Design review of the part built by this model. Coordinates are the model's own, in mm. Coordinates: 2 decimals unless noted, no trailing zeros. Loops run counter-clockwise (first coordinate to the right, second up) from the corner with the lowest first, then second, coordinate; pieces in that order, holes last. Notation, with made-up numbers: (2, 13) - (13, 13) arc R34 cw to (13, 43) - close; hole circle Ø11 at (31, 0.5). An arc over 180 degrees is marked (long way). One line per question, with ' | ' between items.
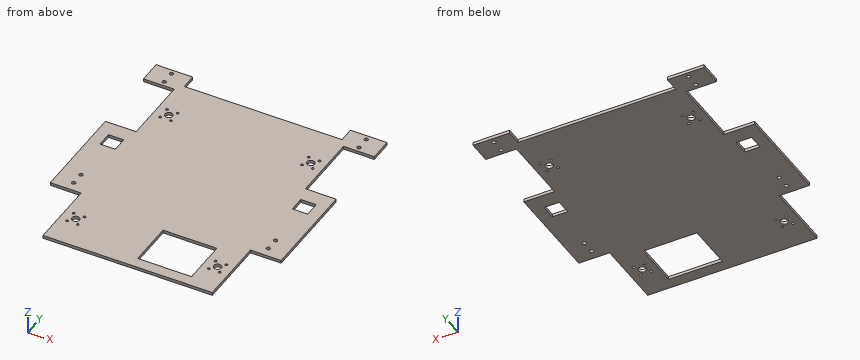
from build123d import *

# Parameters (mm, degrees)
SKETCH_2_R          = 1.65
SKETCH_2_R_2        = 4.9
SKETCH_2_R_3        = 2.5
EXTRUDE_1_DEPTH     = 4
SKETCH_5_W          = 20
SKETCH_5_H          = 20
CUT_EXTRUDE_1_DEPTH = 10
SKETCH_6_W          = 70
SKETCH_6_H          = 60
CUT_EXTRUDE_2_DEPTH = 10


with BuildPart() as part:
    # Sketch 2 → Extrude 1 (new body)
    with BuildSketch(Plane.XY):
        Polygon((40, 0), (260, 0), (260, 90), (300, 90), (300, 220), (260, 220), (260, 310), (300, 310), (300, 340), (252.5, 340), (252.5, 320), (47.5, 320), (47.5, 340), (0, 340), (0, 310), (40, 310), (40, 220), (0, 220), (0, 90), (40, 90), align=None)
        with Locations((50.85, 273)):
            Circle(SKETCH_2_R, mode=Mode.SUBTRACT)
        with Locations((64.85, 273)):
            Circle(SKETCH_2_R, mode=Mode.SUBTRACT)
        with Locations(Location((64.85, 257, 0), (0, 0, 180))):
            Circle(SKETCH_2_R, mode=Mode.SUBTRACT)
        with Locations(Location((50.85, 257, 0), (0, 0, 180))):
            Circle(SKETCH_2_R, mode=Mode.SUBTRACT)
        with Locations((57.8, 265)):
            Circle(SKETCH_2_R_2, mode=Mode.SUBTRACT)
        with Locations((235.15, 257)):
            Circle(SKETCH_2_R, mode=Mode.SUBTRACT)
        with Locations((249.15, 257)):
            Circle(SKETCH_2_R, mode=Mode.SUBTRACT)
        with Locations(Location((242.2, 265, 0), (0, 0, 180))):
            Circle(SKETCH_2_R_2, mode=Mode.SUBTRACT)
        with Locations(Location((235.15, 273, 0), (0, 0, 180))):
            Circle(SKETCH_2_R, mode=Mode.SUBTRACT)
        with Locations(Location((249.15, 273, 0), (0, 0, 180))):
            Circle(SKETCH_2_R, mode=Mode.SUBTRACT)
        with Locations(Location((249.15, 53, 0), (0, 0, 180))):
            Circle(SKETCH_2_R, mode=Mode.SUBTRACT)
        with Locations(Location((235.15, 53, 0), (0, 0, 180))):
            Circle(SKETCH_2_R, mode=Mode.SUBTRACT)
        with Locations((249.15, 37)):
            Circle(SKETCH_2_R, mode=Mode.SUBTRACT)
        with Locations((242.2, 45)):
            Circle(SKETCH_2_R_2, mode=Mode.SUBTRACT)
        with Locations((235.15, 37)):
            Circle(SKETCH_2_R, mode=Mode.SUBTRACT)
        with Locations((50.85, 53)):
            Circle(SKETCH_2_R, mode=Mode.SUBTRACT)
        with Locations((64.85, 53)):
            Circle(SKETCH_2_R, mode=Mode.SUBTRACT)
        with Locations(Location((64.85, 37, 0), (0, 0, 180))):
            Circle(SKETCH_2_R, mode=Mode.SUBTRACT)
        with Locations(Location((57.8, 45, 0), (0, 0, 180))):
            Circle(SKETCH_2_R_2, mode=Mode.SUBTRACT)
        with Locations(Location((50.85, 37, 0), (0, 0, 180))):
            Circle(SKETCH_2_R, mode=Mode.SUBTRACT)
        with Locations((23.5, 333.5)):
            Circle(SKETCH_2_R_3, mode=Mode.SUBTRACT)
        with Locations((23.5, 316.5)):
            Circle(SKETCH_2_R_3, mode=Mode.SUBTRACT)
        with Locations(Location((276.5, 316.5, 0), (0, 0, 180))):
            Circle(SKETCH_2_R_3, mode=Mode.SUBTRACT)
        with Locations(Location((276.5, 333.5, 0), (0, 0, 180))):
            Circle(SKETCH_2_R_3, mode=Mode.SUBTRACT)
        with Locations((23.5, 119.5)):
            Circle(SKETCH_2_R_3, mode=Mode.SUBTRACT)
        with Locations((23.5, 102.5)):
            Circle(SKETCH_2_R_3, mode=Mode.SUBTRACT)
        with Locations(Location((276.5, 102.5, 0), (0, 0, 180))):
            Circle(SKETCH_2_R_3, mode=Mode.SUBTRACT)
        with Locations(Location((276.5, 119.5, 0), (0, 0, 180))):
            Circle(SKETCH_2_R_3, mode=Mode.SUBTRACT)
    extrude(amount=EXTRUDE_1_DEPTH)

    # Sketch 5 → Cut-Extrude 1 (cut)
    with BuildSketch(Plane.XY.offset(4)):
        with Locations((275, 190)):
            Rectangle(SKETCH_5_W, SKETCH_5_H)
        with Locations((25, 190)):
            Rectangle(SKETCH_5_W, SKETCH_5_H)
    extrude(amount=-CUT_EXTRUDE_1_DEPTH, mode=Mode.SUBTRACT)

    # Sketch 6 → Cut-Extrude 2 (cut)
    with BuildSketch(Plane(origin=(0, 0, 0), x_dir=(-1, 0, 0), z_dir=(0, 0, -1))):
        with Locations((-190, 44.5)):
            Rectangle(SKETCH_6_W, SKETCH_6_H)
    extrude(amount=-CUT_EXTRUDE_2_DEPTH, mode=Mode.SUBTRACT)


solid = part.part
Q1. Take a section at C-C (z = 2.55). State how many separate pieces and enclosed holes the cut face has, plus the area to 3 significant figures.
Returned:
separate pieces: 1 | enclosed holes: 31 | area: 77,900 mm²
Q2. Take a section at D-D (y = 245). Give the boundary of the cut face in (x, z), plus the area to 3 significant figures.
Returned:
outline: (40, 0) - (260, 0) - (260, 4) - (40, 4) - close | area: 880 mm²
Q3. Take a section at B-B (x = 216). Give the boundary of the cut face in (y, z), plus the area to 3 significant figures.
Returned:
outline: (0, 0) - (14.5, 0) - (14.5, 4) - (0, 4) - close; (74.5, 0) - (320, 0) - (320, 4) - (74.5, 4) - close | area: 1,040 mm²
Q4. To check wall thickness, follow line 1 along X through (y, z) = (265, 2.75); line 2 along Y through (x, z) = (33, 2.2); line 3 along Y through (x, z) = (57.8, 2.6). State the ranges of each line that lie inside material, in increasing order.
Returned:
line 1: x = 40 to 52.9, 62.7 to 237.3, 247.1 to 260 | line 2: y = 90 to 180, 200 to 220, 310 to 340 | line 3: y = 0 to 40.1, 49.9 to 260.1, 269.9 to 320
Q5. For pin 1 (1.5 mm diameter, centred on x = 214, z = 1.5, fed in from -Y); pin 2 (1.2 mm diameter, centred on x = 14, z = 3, fed in from -Y); pin 3 (2 mm diameter, centred on y = 260.5, z = 2.5, fed in from +X), all flat-tipped, find the tip position at first contact; note any pin that passes through.
Returned:
pin 1: stops at y = 0 | pin 2: stops at y = 90 | pin 3: stops at x = 260
Q6. Take a section at A-A (y = 29). Give the boundary of the cut face in (x, z).
Returned:
outline: (40, 0) - (155, 0) - (155, 4) - (40, 4) - close; (225, 0) - (260, 0) - (260, 4) - (225, 4) - close
